Build history of the part. All positions in model axes, mm. Face numbers are marked on the shaded views. A direction names the side the tool comes from. Give positions to 0.01 mm unless a question says otherwise; leave off trailing zeros. Order: outer loops, then holes, each group sorted by start corner. A loop starts at its lowest first (then second) coordinate and runs counter-clockwise, first axis right, second up. Notation, with made-up numbers: M -30,17 L 23,17 A26 ccw 23,47 Z; hole C 1,38 d9. An arc over 180 degrees is marked long. One line per item, written item: value.
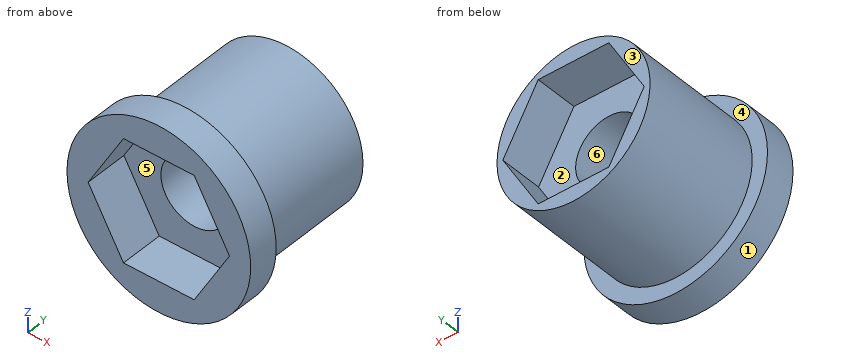
Autodesk Inventor part; units mm, degrees
ref_plane "YZ Plane" through (0, 0, 0) normal (1, 0, 0) x (0, 1, 0)
ref_plane "XZ Plane" through (0, 0, 0) normal (0, 1, 0) x (-1, 0, 0)
ref_plane "XY Plane" through (0, 0, 0) normal (0, 0, 1) x (1, 0, 0)
sketch "Эскиз1" plane through (0, 0, 0) normal (0, 1, 0) x (-1, 0, 0)
  circle A0 centre (0, 0) radius 3
  dimension "d0" = 6
extrude "Выдавливание1" add sketch "Эскиз1" along normal blind 1
sketch "Эскиз2" plane through (0, 1, 0) normal (0, 1, 0) x (1, 0, 0)
  circle A0 centre (0, 0) radius 2.5
  dimension "d3" = 5
extrude "Выдавливание2" add sketch "Эскиз2" along normal blind 4
sketch "Эскиз3" plane through (0, 5, 0) normal (0, 1, 0) x (1, 0, 0)
  circle A0 centre (0, 0) radius 3
  line L0 (-2.3094, 0) -> (-1.1547, 2)
  line L1 (-1.1547, 2) -> (1.1547, 2)
  line L2 (1.1547, 2) -> (2.3094, 0)
  line L3 (2.3094, 0) -> (1.1547, -2)
  line L4 (1.1547, -2) -> (-1.1547, -2)
  line L5 (-1.1547, -2) -> (-2.3094, 0)
  dimension "d6" = 4
extrude "Выдавливание3" cut sketch "Эскиз3" against normal blind 1.4 contours L0 L1 L2 L3 L4 L5
sketch "Эскиз4" plane through (0, 3.6, 0) normal (0, 1, 0) x (1, 0, 0)
  circle A0 centre (0, 0) radius 1.1
  dimension "d9" = 2.2
extrude "Выдавливание4" cut sketch "Эскиз4" against normal up to surface (3.6 mm away)
sketch "Эскиз5" plane through (0, 0, 0) normal (0, -1, 0) x (1, 0, 0)
  line L0 (2.3094, 0) -> (1.1547, -2)
  line L1 (1.1547, -2) -> (-1.1547, -2)
  line L2 (-1.1547, -2) -> (-2.3094, 0)
  line L3 (-2.3094, 0) -> (-1.1547, 2)
  line L4 (-1.1547, 2) -> (1.1547, 2)
  line L5 (1.1547, 2) -> (2.3094, 0)
  point P0 (0, 0)
  point P1 (0, 0)
  dimension "d12" = 4
extrude "Выдавливание5" cut sketch "Эскиз5" against normal blind 1.4
properties part number "втулка_каретка"
1) Mould opens along Z. For the marked faces 1, 2 and 3 say: released by +Z, released by -Z, zero draft, split by the parting line, or undercut.
Check values:
face 1: split by the parting line
face 2: undercut
face 3: zero draft
2) Saw through at A-A, the plane y = 0.7. Write the cut outline in (x, z), then the cut area to 3 significant figures.
Check values:
outline: C 0,0 d6; hole M -2.31,0 L -1.15,-2 L 1.15,-2 L 2.31,0 L 1.15,2 L -1.15,2 Z
area: 14.4 mm^2
3) Saw through at D-D, the plane z = -1.9. Write the cut outline in (x, y).
Check values:
outline: M -2.32,0 L -1.21,0 L -1.21,1.4 L 1.21,1.4 L 1.21,0 L 2.32,0 L 2.32,1 L 1.62,1 L 1.62,5 L 1.21,5 L 1.21,3.6 L -1.21,3.6 L -1.21,5 L -1.62,5 L -1.62,1 L -2.32,1 Z
4) Pin check, flat tips, straight feed: pin 1 (1.1 mm diameter, centred on x = 0, y = 4.5, fed in from -Z); pin 2 (3 mm diameter, centred on x = 0, z = 0, fed in from +Y); pin 3 (0.7 mm diameter, centred on x = 0, y = 4.5, fed in from +Z). Stop position of each tip, or through.
Check values:
pin 1: z = -2.5
pin 2: y = 3.6
pin 3: z = 2.5
5) Tool access for the marked faces 4, 5 and 6: list every direction of +Z, -Z, +X, -X, +Y, -Y with a clear straight run to the whole face (end or side of a thin tool).
Check values:
face 4: +Y
face 5: -Y
face 6: +Y, -Y
6) Drill centre lines: probe 1 along X at (y, z) = (1.9, 0); probe 2 along Z at (x, y) = (-0.1, 0.5). Where is each one in solid material? Low to high. Write a range as from..to.
Check values:
probe 1: -2.5..-1.1, 1.1..2.5
probe 2: -3..-2, 2..3
7) Saw through at C-C, the plane z = 0.7. Write the cut outline in (x, y).
Check values:
outline: M -2.92,0 L -1.91,0 L -1.91,1.4 L -0.85,1.4 L -0.85,3.6 L -1.91,3.6 L -1.91,5 L -2.4,5 L -2.4,1 L -2.92,1 Z; M 0.85,1.4 L 1.91,1.4 L 1.91,0 L 2.92,0 L 2.92,1 L 2.4,1 L 2.4,5 L 1.91,5 L 1.91,3.6 L 0.85,3.6 Z
8) Saw through at B-B, the plane x = 0. Write the cut outline in (y, z).
Check values:
outline: M 0,-3 L 1,-3 L 1,-2.5 L 5,-2.5 L 5,-2 L 3.6,-2 L 3.6,-1.1 L 1.4,-1.1 L 1.4,-2 L 0,-2 Z; M 0,2 L 1.4,2 L 1.4,1.1 L 3.6,1.1 L 3.6,2 L 5,2 L 5,2.5 L 1,2.5 L 1,3 L 0,3 Z
